Input: dimensioned drawing with shaded views. Units: mm. Origin: part minimum x, y, z. Round coordinates to 2 decimals unless told otherwise and drop trailing zeros. Loops run counter-clockwise (first coordinate to the right, second up) from the corner with the lowest first, then second, coordinate; pieces in that order, holes last. Notation, with made-up numbers: M -1.5,-9.5 L 10.5,-9.5 A14 cw 10.5,0.5 Z; hole C 64.5,-23.75 d9. An arc over 180 degrees is marked long. Use one line per item in the form item = value. Start each with the question number.
Q1. Section query A-A, the plane z = 36.5. Output: boundary loops of the cut face in (x, y), and give its area (3 significant figures).
Q2. First-contact query: P1, Ø3.5, axis at x = 21.5, z = 57.75, coming from the -Y side. Flat tip, straight axial feed; report the tip coordinate or a pass-through.
Q3. Section query C-C, the plane y = 0.25. Output: boundary loops of the cut face in (x, z), and give its area (3 significant figures).
Q4. Section query D-D, the plane x = 26.5. Output: boundary loops of the cut face in (y, z), and give its area (3 significant figures).
Q5. Ray query, line 1 along Z through (x, y) = (21.5, 0.85); line 2 along Z through (x, y) = (12, 0.4); line 3 along X through (y, z) = (1, 7.25). Return the intervals inside material, ascending.
Q6. Section query B-B, the plane x = 21.5. Output: boundary loops of the cut face in (y, z), and give its area (3 significant figures).
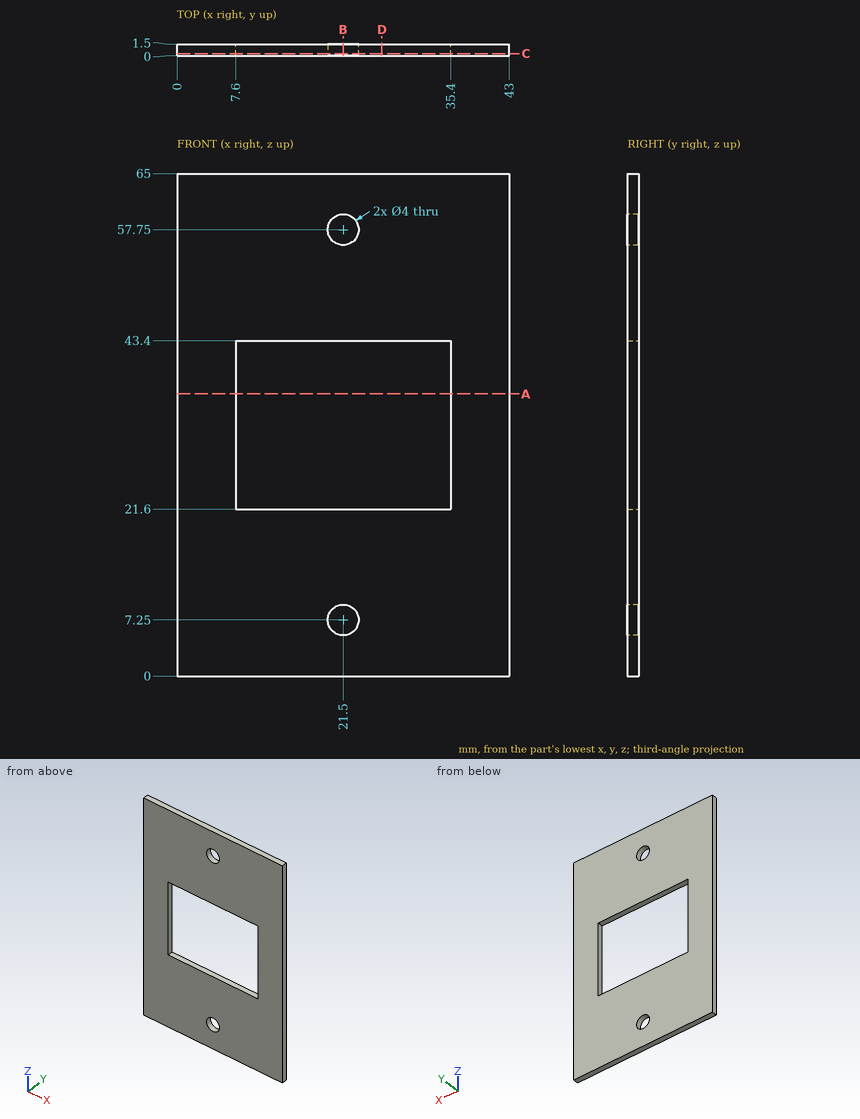
Results found:
q1.outline = M 0,0 L 7.6,0 L 7.6,1.5 L 0,1.5 Z; M 35.4,0 L 43,0 L 43,1.5 L 35.4,1.5 Z
q1.area = 22.8 mm²
q2.P1 = through
q3.outline = M 0,0 L 43,0 L 43,65 L 0,65 Z; hole M 7.6,21.6 L 35.4,21.6 L 35.4,43.4 L 7.6,43.4 Z; hole C 21.5,7.25 d4; hole C 21.5,57.75 d4
q3.area = 2,160 mm²
q4.outline = M 0,0 L 1.5,0 L 1.5,21.6 L 0,21.6 Z; M 0,43.4 L 1.5,43.4 L 1.5,65 L 0,65 Z
q4.area = 64.8 mm²
q5.line_1 = 0 to 5.25, 9.25 to 21.6, 43.4 to 55.75, 59.75 to 65
q5.line_2 = 0 to 21.6, 43.4 to 65
q5.line_3 = 0 to 19.5, 23.5 to 43
q6.outline = M 0,0 L 1.5,0 L 1.5,5.25 L 0,5.25 Z; M 0,9.25 L 1.5,9.25 L 1.5,21.6 L 0,21.6 Z; M 0,43.4 L 1.5,43.4 L 1.5,55.75 L 0,55.75 Z; M 0,59.75 L 1.5,59.75 L 1.5,65 L 0,65 Z
q6.area = 52.8 mm²
